Part model, mm, in its own coordinate system. Face numbers are marked on the shaded views. Round coordinates to 2 decimals unless told otherwise and drop trailing zeros. Loops run counter-clockwise (first coordinate to the right, second up) from the corner with the lowest first, then second, coordinate; pieces in that order, holes last. Notation, with made-up numbers: (20.5, -11) - (46.5, -11) arc R34 cw to (46.5, 24) - close; hole circle Ø7 at (-21.75, 44). An arc over 180 degrees is marked (long way). Put each result on its own line as item: value.
from build123d import *

# Parameters (mm, degrees)
SKETCH1_W           = 98
SKETCH1_H           = 98
BOSS_EXTRUDE1_DEPTH = 10
SKETCH8_W           = 98
SKETCH8_H           = 98
SKETCH8_W_2         = 78
SKETCH8_H_2         = 78
CUT_EXTRUDE5_DEPTH  = 5
SKETCH14_R          = 1.5
CUT_EXTRUDE11_DEPTH = 10
SKETCH15_W          = 10
SKETCH15_H          = 20
CUT_EXTRUDE19_DEPTH = 10
FILLET1_R           = 2


with BuildPart() as part:
    # Sketch1 → Boss-Extrude1 (new body)
    with BuildSketch(Plane(origin=(0, 0, 0), x_dir=(1, 0, 0), z_dir=(0, 1, 0))):
        Rectangle(SKETCH1_W, SKETCH1_H)
    extrude(amount=BOSS_EXTRUDE1_DEPTH)

    # Sketch8 → Cut-Extrude5 (cut)
    with BuildSketch(Plane(origin=(0, 10, 0), x_dir=(1, 0, 0), z_dir=(0, 1, 0))):
        Rectangle(SKETCH8_W, SKETCH8_H)
        Rectangle(SKETCH8_W_2, SKETCH8_H_2, mode=Mode.SUBTRACT)
    extrude(amount=-CUT_EXTRUDE5_DEPTH, mode=Mode.SUBTRACT)

    # Sketch14 → Cut-Extrude11 (cut)
    with BuildSketch(Plane.XZ):
        with Locations(Location((-44, -44, 0), (0, 0, 270))):
            Circle(SKETCH14_R)
        with Locations(Location((-44, 44, 0), (0, 0, 270))):
            Circle(SKETCH14_R)
        with Locations(Location((44, 44, 0), (0, 0, 270))):
            Circle(SKETCH14_R)
        with Locations(Location((44, -44, 0), (0, 0, 270))):
            Circle(SKETCH14_R)
    extrude(amount=-CUT_EXTRUDE11_DEPTH, mode=Mode.SUBTRACT)

    # Sketch15 → Cut-Extrude19 (cut)
    with BuildSketch(Plane(origin=(0, 10, 0), x_dir=(1, 0, 0), z_dir=(0, 1, 0))):
        with BuildLine():
            ThreePointArc((-34, 32), (-33.414213562, 33.414213562), (-32, 34))
            Line((-32, 34), (32, 34))
            ThreePointArc((32, 34), (33.414213562, 33.414213562), (34, 32))
            Line((34, 32), (34, 31))
            ThreePointArc((34, 31), (33.414213562, 29.585786438), (32, 29))
            Line((32, 29), (14, 29))
            Line((14, 29), (-14, 29))
            Line((-14, 29), (-32, 29))
            ThreePointArc((-32, 29), (-33.414213562, 29.585786438), (-34, 31))
            Line((-34, 31), (-34, 32))
        make_face()
        with BuildLine():
            ThreePointArc((-34, 21.5), (-33.414213562, 22.914213562), (-32, 23.5))
            Line((-32, 23.5), (-14, 23.5))
            Line((-14, 23.5), (14, 23.5))
            Line((14, 23.5), (32, 23.5))
            ThreePointArc((32, 23.5), (33.414213562, 22.914213562), (34, 21.5))
            Line((34, 21.5), (34, 20.5))
            ThreePointArc((34, 20.5), (33.414213562, 19.085786438), (32, 18.5))
            Line((32, 18.5), (14, 18.5))
            Line((14, 18.5), (-14, 18.5))
            Line((-14, 18.5), (-32, 18.5))
            ThreePointArc((-32, 18.5), (-33.414213562, 19.085786438), (-34, 20.5))
            Line((-34, 20.5), (-34, 21.5))
        make_face()
        with BuildLine():
            ThreePointArc((-19, 11), (-18.414213562, 12.414213562), (-17, 13))
            Line((-17, 13), (-14, 13))
            Line((-14, 13), (14, 13))
            Line((14, 13), (17, 13))
            ThreePointArc((17, 13), (18.414213562, 12.414213562), (19, 11))
            Line((19, 11), (19, 10))
            ThreePointArc((19, 10), (18.414213562, 8.585786438), (17, 8))
            Line((17, 8), (14, 8))
            Line((14, 8), (-14, 8))
            Line((-14, 8), (-17, 8))
            ThreePointArc((-17, 8), (-18.414213562, 8.585786438), (-19, 10))
            Line((-19, 10), (-19, 11))
        make_face()
        with BuildLine():
            ThreePointArc((-19, 0.5), (-18.414213562, 1.914213562), (-17, 2.5))
            Line((-17, 2.5), (-14, 2.5))
            Line((-14, 2.5), (14, 2.5))
            Line((14, 2.5), (17, 2.5))
            ThreePointArc((17, 2.5), (18.414213562, 1.914213562), (19, 0.5))
            Line((19, 0.5), (19, -0.5))
            ThreePointArc((19, -0.5), (18.414213562, -1.914213562), (17, -2.5))
            Line((17, -2.5), (14, -2.5))
            Line((14, -2.5), (-14, -2.5))
            Line((-14, -2.5), (-17, -2.5))
            ThreePointArc((-17, -2.5), (-18.414213562, -1.914213562), (-19, -0.5))
            Line((-19, -0.5), (-19, 0.5))
        make_face()
        with BuildLine():
            ThreePointArc((-19, -10), (-18.414213562, -8.585786438), (-17, -8))
            Line((-17, -8), (-14, -8))
            Line((-14, -8), (14, -8))
            Line((14, -8), (17, -8))
            ThreePointArc((17, -8), (18.414213562, -8.585786438), (19, -10))
            Line((19, -10), (19, -11))
            ThreePointArc((19, -11), (18.414213562, -12.414213562), (17, -13))
            Line((17, -13), (14, -13))
            Line((14, -13), (-14, -13))
            Line((-14, -13), (-17, -13))
            ThreePointArc((-17, -13), (-18.414213562, -12.414213562), (-19, -11))
            Line((-19, -11), (-19, -10))
        make_face()
        with BuildLine():
            ThreePointArc((32, -18.5), (33.414213562, -19.085786438), (34, -20.5))
            Line((34, -20.5), (34, -21.5))
            ThreePointArc((34, -21.5), (33.414213562, -22.914213562), (32, -23.5))
            Line((32, -23.5), (14, -23.5))
            Line((14, -23.5), (-14, -23.5))
            Line((-14, -23.5), (-32, -23.5))
            ThreePointArc((-32, -23.5), (-33.414213562, -22.914213562), (-34, -21.5))
            Line((-34, -21.5), (-34, -20.5))
            ThreePointArc((-34, -20.5), (-33.414213562, -19.085786438), (-32, -18.5))
            Line((-32, -18.5), (-14, -18.5))
            Line((-14, -18.5), (14, -18.5))
            Line((14, -18.5), (32, -18.5))
        make_face()
        with BuildLine():
            ThreePointArc((32, -29), (33.414213562, -29.585786438), (34, -31))
            Line((34, -31), (34, -32))
            ThreePointArc((34, -32), (33.414213562, -33.414213562), (32, -34))
            Line((32, -34), (-32, -34))
            ThreePointArc((-32, -34), (-33.414213562, -33.414213562), (-34, -32))
            Line((-34, -32), (-34, -31))
            ThreePointArc((-34, -31), (-33.414213562, -29.585786438), (-32, -29))
            Line((-32, -29), (-14, -29))
            Line((-14, -29), (14, -29))
            Line((14, -29), (32, -29))
        make_face()
        with Locations((-29, 0)):
            Rectangle(SKETCH15_W, SKETCH15_H)
        with Locations((29, 0)):
            Rectangle(SKETCH15_W, SKETCH15_H)
    extrude(amount=-CUT_EXTRUDE19_DEPTH, mode=Mode.SUBTRACT)

    # Fillet1
    fillet1_edges = [part.edges().sort_by_distance(p)[0] for p in [
        (34, 5, -10),
        (34, 5, 10),
        (24, 5, 10),
        (24, 5, -10),
        (-34, 5, -10),
        (-24, 5, -10),
        (-24, 5, 10),
        (-34, 5, 10),
    ]]
    fillet(fillet1_edges, radius=FILLET1_R)


solid = part.part
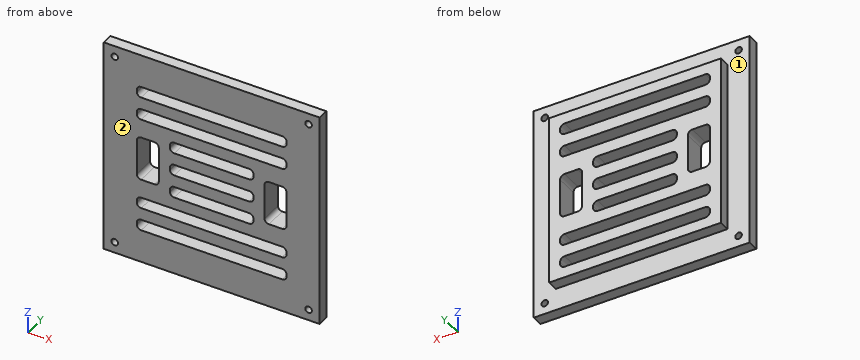
1. Pin check, flat tips, straight feed: P1, Ø2, axis at y = 9, z = -18.5, coming from the +X side; P2, Ø1.8, axis at x = -44, z = -44, coming from the +Y side; P3, Ø3, axis at x = -14, y = 5.5, coming from the +Z side; P4, Ø1.5, axis at y = 8.5, z = -21, coming from the -X side. Stop position of each tip, or through.
A:
P1: stops at x = 39
P2: passes through
P3: stops at z = 49
P4: stops at x = -39
2. Probe line 1 along X through (y, z) = (1.8, -44); line 2 along Z through (x, y) = (28, 1.5); line 3 along Z through (x, y) = (26, 7.25). List the from-to ranges inside material, lowest first. Write a range as [from, to].
A:
line 1: x = [-49, -45.5], [-42.5, 42.5], [45.5, 49]
line 2: z = [-49, -34], [-29, -23.5], [-18.5, -10], [10, 18.5], [23.5, 29], [34, 49]
line 3: z = [-39, -34], [-29, -23.5], [-18.5, -10], [10, 18.5], [23.5, 29], [34, 39]
3. Band-saw the part on C-C (x = -44). List the corners of the cut face in (y, z).
A:
outline: (0, -49) - (5, -49) - (5, -45.5) - (0, -45.5) - close; (0, -42.5) - (5, -42.5) - (5, 42.5) - (0, 42.5) - close; (0, 45.5) - (5, 45.5) - (5, 49) - (0, 49) - close
4. Band-saw the part on B-B (z = 5.5). List the corners of the cut face in (x, y), plus the area to 3 significant figures.
A:
outline: (-49, 0) - (-34, 0) - (-34, 10) - (-39, 10) - (-39, 5) - (-49, 5) - close; (-24, 0) - (24, 0) - (24, 10) - (-24, 10) - close; (34, 0) - (49, 0) - (49, 5) - (39, 5) - (39, 10) - (34, 10) - close
area: 680 mm²
5. Band-saw the part on A-A (x = 28). List the corners of the cut face in (y, z).
A:
outline: (0, -49) - (5, -49) - (5, -39) - (10, -39) - (10, -34) - (0, -34) - close; (0, -29) - (10, -29) - (10, -23.5) - (0, -23.5) - close; (0, -18.5) - (10, -18.5) - (10, -10) - (0, -10) - close; (0, 10) - (10, 10) - (10, 18.5) - (0, 18.5) - close; (0, 23.5) - (10, 23.5) - (10, 29) - (0, 29) - close; (0, 34) - (10, 34) - (10, 39) - (5, 39) - (5, 49) - (0, 49) - close
6. Two-plate mould, pull along Y, no slides. Class the marked faces 1 and 2: pulls with the +Y half, pulls with the -Y half, needs draft (parallel to the pull), parting line crosses it, or undercut.
A:
face 1: pulls with the +Y half
face 2: pulls with the -Y half
7. Band-saw the part on D-D (y = 6.75). Give the number of separate pieces and of enclosed holes in the cut face, plus the area to 3 significant figures.
A:
separate pieces: 1
enclosed holes: 9
area: 3,780 mm²
